from build123d import *

# Parameters (mm, degrees)
F1_DEPTH = 2.54
F2_SCALE = 1.12
F3_R     = 1.27
F4_R     = 2.2098
F5_DEPTH = 7.0104
F6_ANGLE = 180
F7_DEPTH = 1.27
F8_R     = 5.1308
F8_R_2   = 2.2098
F9_DEPTH = 1.27


with BuildPart() as f1:
    # F0 (on Top) → F1 (new body)
    with BuildSketch(Plane.XY):
        Polygon((2.6097216178, 14.5627437159), (-2.4016266689, 14.6046923473), (-2.4016266689, 10.7069099322), (-6.7973635159, 8.6464090273), (-9.7507489845, 11.1018400639), (-12.9371215583, 7.269280193), (-9.9187448393, 4.759815731), (-10.987800546, 0.1461525389), (-14.7898914292, -0.6685812259), (-13.7329729143, -5.6008676039), (-9.9187448393, -4.7835330123), (-6.9650523365, -8.5103949532), (-8.662414737, -11.9730141014), (-4.136644538, -14.1915290003), (-2.4166579341, -10.6827564792), (2.3025460541, -10.6827564792), (3.9659612812, -14.2644541338), (8.5153820935, -12.1516080526), (6.8819414162, -8.6344521752), (9.8897544667, -4.8440932296), (13.6239528656, -5.7776425965), (14.7675592452, -0.8934023208), (10.9942825511, -0.0382388607), (9.9505092949, 4.6697063372), (13.008704409, 7.0334360935), (9.9016642198, 10.9836040065), (6.8838195875, 8.5752755404), (2.5481330231, 10.6975259259), align=None)
    extrude(amount=F1_DEPTH)


with BuildPart() as f1_1:
    # F2: moved
    add(f1.part.scale(F2_SCALE))

    # F3
    f3_edges = [f1_1.edges().sort_by_distance(p)[0] for p in [
        (-16.564678, -0.748811, 1.4224),
        (-12.306337, 0.163691, 1.4224),
        (-14.489576, 8.141594, 1.4224),
        (-10.920839, 12.434061, 1.4224),
        (-7.613047, 9.683978, 1.4224),
        (-2.689822, 11.991739, 1.4224),
        (-2.689822, 16.357255, 1.4224),
        (2.922888, 16.310273, 1.4224),
        (2.853909, 11.981229, 1.4224),
        (7.709878, 9.604309, 1.4224),
        (11.089864, 12.301636, 1.4224),
        (14.569749, 7.877448, 1.4224),
        (11.14457, 5.230071, 1.4224),
        (12.313596, -0.042828, 1.4224),
        (16.539666, -1.000611, 1.4224),
        (15.258827, -6.47096, 1.4224),
        (11.076525, -5.425384, 1.4224),
        (7.707774, -9.670586, 1.4224),
        (9.537228, -13.609801, 1.4224),
        (4.441877, -15.976189, 1.4224),
        (2.578852, -11.964687, 1.4224),
        (-2.706657, -11.964687, 1.4224),
        (-4.633042, -15.894512, 1.4224),
        (-9.701905, -13.409776, 1.4224),
        (-7.800859, -9.531642, 1.4224),
        (-11.108994, -5.357557, 1.4224),
        (-15.38093, -6.272972, 1.4224),
        (-11.108994, 5.330994, 1.4224),
    ]]
    fillet(f3_edges, radius=F3_R)

    # F4 (on face) → F5 (join)
    with BuildSketch(Plane.XY):
        Circle(F4_R)
    extrude(amount=-F5_DEPTH)


with BuildPart() as f1_2:
    # F6: moved
    add(f1_1.part.rotate(Axis((-0.0732200051, -11.9646872567, 0), (1, 0, 0)), F6_ANGLE))

    # F7 (cut): a face of the model
    f7_faces = [f1_2.faces().sort_by_distance(p)[0] for p in [
        (5.0824398182, -34.3118398385, 0),
    ]]
    extrude(f7_faces, amount=-F7_DEPTH, mode=Mode.SUBTRACT)

    # F8 (on face) → F9 (join)
    with BuildSketch(Plane.XY.offset(-1.27)):
        with Locations((0, -23.9293745135)):
            Circle(F8_R)
        with Locations((0, -23.9293745135)):
            Circle(F8_R_2, mode=Mode.SUBTRACT)
    extrude(amount=F9_DEPTH)


solid = f1_2.part
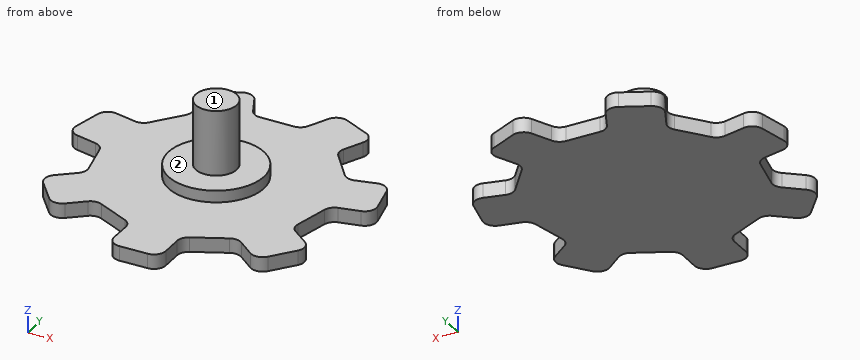
Verification items for the finished model (mm, model axes). Face numbers are marked on the shaded views. A direction names the side the tool comes from. Coordinates: 2 decimals unless noted, no trailing zeros. Order: outer loops, then holes, each group sorted by start corner. A loop starts at its lowest first (then second) coordinate and runs counter-clockwise, first axis right, second up.
1. Sectioned sample at B-B, the plane x = -0.5. Record the cut outline in (y, z), and give its area (3 significant figures).
Results found:
outline: (-40.27, -2.84) - (-11.96, -2.84) - (-11.96, -1.27) - (-18.82, -1.27) - (-18.82, 0) - (-21.78, 0) - (-21.78, 7.01) - (-26.08, 7.01) - (-26.08, 0) - (-29.04, 0) - (-29.04, -1.27) - (-40.27, -1.27) - close
area: 87.7 mm2
2. Sectioned sample at C-C, the plane z = 4.25. Record the cut outline in (x, y).
Results found:
outline: circle Ø4.42 at (0, -23.93)
3. Go/stop test with flat-tipped pins: pin 1 Ø0.8 at (y, z) = (-38, -2.5) entering from -X; pin 2 Ø0.5 at (x, z) = (-1, -2.5) entering from +Y; pin 3 Ø10 at (x, y) = (-11.5, -31) entering from +Z. Record where each tip stops, or that it passes through.
Results found:
pin 1: stops at x = -2.69
pin 2: stops at y = -11.96
pin 3: stops at z = -1.27
4. Scan lines: line 1 (Z direction, x = 7, y = -11); line 2 (Y direction, x = 2, z = -2); line 3 (Y direction, x = -4, z = -2.5). Record each from-to range of solid material in increasing order.
Results found:
line 1: z = -2.84 to -1.27
line 2: y = -40.2 to -11.94
line 3: y = -35.31 to -9.33
5. Set-up check for the marked faces 1 and 2: record each of +Z, -Z, +X, -X, +Y, -Y from which the full face is reachable in a straight line by a thin tool's end or side.
Results found:
face 1: +Z, +X, -X, +Y, -Y
face 2: +Z
6. Sectioned sample at A-A, the plane y = -27. Record the cut outline in (x, z), and give its area (3 significant figures).
Results found:
outline: (-11.63, -2.84) - (11.62, -2.84) - (11.62, -1.27) - (4.11, -1.27) - (4.11, 0) - (-4.11, 0) - (-4.11, -1.27) - (-11.63, -1.27) - close
area: 47.1 mm2
7. Sectioned sample at D-D, the plane y = -15.5. Record the cut outline in (x, z).
Results found:
outline: (-8.67, -2.84) - (8.69, -2.84) - (8.69, -1.27) - (-8.67, -1.27) - close
